Geometry check sheet. Reference: the model listing, model coordinates, mm. Face numbers are marked on the shaded views. A direction names the side the tool comes from. Give positions to 0.01 mm unless a question says otherwise; leave off trailing zeros. Write each loop counter-clockwise with the first axis right and the second up, starting at its lowest first coordinate (ties: lowest second). Pieces come first, ordered by that corner, then holes. Notation, with made-up numbers: (80.5, 22) - (123.5, 22) arc R20 ccw to (123.5, 54) - close; hole circle Ø9 at (55, -27). An arc over 180 degrees is marked (long way). Write item = value, one per line. Start each with the question number.
(1) Section check C-C, the plane y = 19.5. Enter the section's corners in (x, z) (3 decimals).
(2) Section check A-A, the plane z = 0.55. Enter the section's corners in (x, y).
(3) Thickness scan on L1, parallel to Y at x = -2.5, z = 0.4; L2, parallel to X at y = 18, z = 0.7; L3, parallel to Z at x = -11.5, y = 15.25 (3 decimals). Record the ranges inside material, lowest first.
(4) Draft check along X on the marked faces 4, 5, 6 and 7. Enter one of: pulls with the +X half, pulls with the -X half, needs draft (parallel to the pull), parting line crosses it, or undercut.
(5) Depth check by flat-ended pin: pin 1 Ø1.3 at (x, y) = (-12, 18.5) entering from -Z; pin 2 Ø3 at (x, y) = (-4.5, 21) entering from +Z. Enter the tip coordinate at first touch or a pass-through.
(6) Section check B-B, the plane x = -7.5. Enter the section's corners in (y, z) (3 decimals).
(7) Access from +Z, -Z, +X, -X, +Y, -Y to the whole of each face (thin tool, end or side, straight path). Record for the marked faces 1, 2 and 3.
(8) Section check D-D, the plane z = 2.9. Enter the section's corners in (x, y), plus the area to 3 significant figures.
```python
from build123d import *

# Parameters (mm, degrees)
F0_W     = 15.9004
F0_H     = 7.9502
F0_R     = 2.3876
F1_DEPTH = 3.175
F2_DEPTH = 4.7752
F3_T     = -1.6002


with BuildPart() as f1:
    # F0 (on Top) → F1 (new body)
    with BuildSketch(Plane.XY):
        with Locations((-7.9505280386, 18.2070285082)):
            Rectangle(F0_W, F0_H)
        with Locations((-11.9383280386, 18.2197285082)):
            Circle(F0_R, mode=Mode.SUBTRACT)
        with Locations((-3.9881280386, 18.2197285082)):
            Circle(F0_R, mode=Mode.SUBTRACT)
    extrude(amount=F1_DEPTH)

    # F0 (on Top) → F2 (join)
    with BuildSketch(Plane.XY):
        with Locations((-11.9383280386, 18.2197285082)):
            Circle(F0_R)
        with Locations((-3.9881280386, 18.2197285082)):
            Circle(F0_R)
    extrude(amount=F2_DEPTH)

    # F3
    f3_openings = [f1.faces().sort_by_distance(p)[0] for p in [
        (-7.950528, 18.207029, 0),
    ]]
    offset(amount=F3_T, openings=f3_openings, kind=Kind.INTERSECTION)


solid = f1.part
```
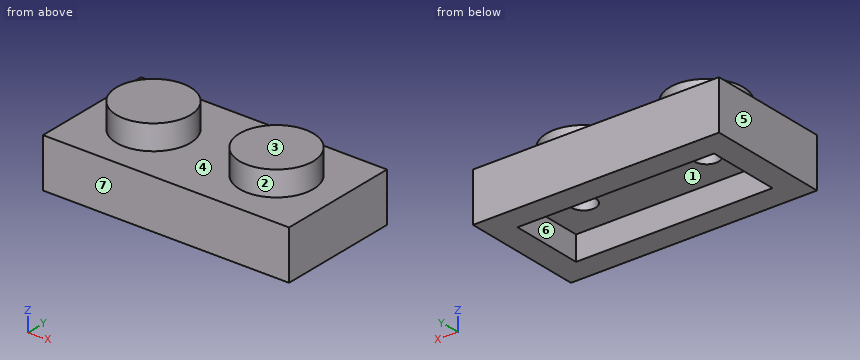
Model answer:
q1.outline = (-15.901, 0) - (-14.301, 0) - (-14.301, 1.575) - (-1.601, 1.575) - (-1.601, 0) - (0, 0) - (0, 3.175) - (-1.973, 3.175) - (-1.973, 4.775) - (-6.003, 4.775) - (-6.003, 3.175) - (-9.923, 3.175) - (-9.923, 4.775) - (-13.954, 4.775) - (-13.954, 3.175) - (-15.901, 3.175) - close
q2.outline = (-15.9, 14.23) - (0, 14.23) - (0, 22.18) - (-15.9, 22.18) - close; hole (-14.3, 15.83) - (-1.6, 15.83) - (-1.6, 20.58) - (-14.3, 20.58) - close
q3.L1 = 14.23 to 15.83, 20.58 to 22.18
q3.L2 = -15.9 to -14.3, -1.6 to 0
q3.L3 = 0 to 3.175
q4.face_4 = undercut
q4.face_5 = pulls with the -X half
q4.face_6 = undercut
q4.face_7 = needs draft
q5.pin_1 = 1.57
q5.pin_2 = 4.78
q6.outline = (14.232, 0) - (15.832, 0) - (15.832, 1.575) - (20.582, 1.575) - (20.582, 0) - (22.182, 0) - (22.182, 3.175) - (14.232, 3.175) - close
q7.face_1 = -Z
q7.face_2 = +Z
q7.face_3 = +Z, +X, -X, +Y, -Y
q8.outline = (-15.9, 14.23) - (0, 14.23) - (0, 22.18) - (-15.9, 22.18) - close; hole circle Ø1.57 at (-11.94, 18.22); hole circle Ø1.57 at (-3.99, 18.22)
q8.area = 123 mm²
